Model file for the job. Use its own axes, mm. A direction names the side the tool comes from. Coordinates: 2 decimals unless noted, no trailing zeros. Order: outer loops, then holes, each group sorted by start corner. A loop starts at its lowest first (then second) coordinate and runs counter-clockwise, first axis right, second up.
from build123d import *

# Parameters (mm, degrees)
THICKNESS_EXTRUDE_DEPTH = 2
HOOK_1_EXTRUDE_DEPTH    = 0.9
HOOK_START              = -26.75
HOOK_2_EXTRUDE_DEPTH    = 0.9
HOOK_PATTERN_COUNT      = 2
HOOK_PATTERN_PITCH      = 96


with BuildPart() as part:
    # Top Sketch → Thickness Extrude (new body)
    with BuildSketch(Plane(origin=(0, 0, 0), x_dir=(1, 0, 0), z_dir=(0, 1, 0))):
        Polygon((-28, -21.5), (-28, -22.875), (-31, -22.875), (-31, -21.5), (-124, -21.5), (-124, -22.875), (-127, -22.875), (-127, -21.5), (-168, -21.5), (-168, 0), (-127, 0), (-127, 3.875), (-124, 3.875), (-124, 0), (-31, 0), (-31, 3.875), (-28, 3.875), (-28, 0), (0, 0), (0, -21.5), align=None)
    extrude(amount=THICKNESS_EXTRUDE_DEPTH)


with BuildPart() as body_2:
    # Hook Sketch → Hook 1 Extrude (new, symmetric)
    with BuildSketch(Plane.XY.offset(22.875)):
        Polygon((-31, 2), (-28, 2), (-28, -4.258262488), (-36, -4.258262488), (-36, -2.258262488), (-31, -1.6), align=None)
    hook_1_extrude = extrude(amount=HOOK_1_EXTRUDE_DEPTH, both=True)


with BuildPart() as body_3:
    # Hook Sketch<2> → Hook 2 Extrude (new, symmetric)
    with BuildSketch(Plane.XY.offset(22.875).offset(HOOK_START)):
        Polygon((-31, 2), (-28, 2), (-28, -4.258262488), (-36, -4.258262488), (-36, -2.258262488), (-31, -1.6), align=None)
    hook_2_extrude = extrude(amount=HOOK_2_EXTRUDE_DEPTH, both=True)


with BuildPart() as hook_pattern_1:
    # Hook Pattern: pattern copy
    add(hook_1_extrude.moved(Location(Vector(-1, 0, 0) * (1 * HOOK_PATTERN_PITCH))))


with BuildPart() as hook_pattern_2:
    # Hook Pattern: pattern copy
    add(hook_2_extrude.moved(Location(Vector(-1, 0, 0) * (1 * HOOK_PATTERN_PITCH))))


with BuildPart() as part_1:
    add(part.part)

    # Combine Bodies: union body 2, body 3, Hook Pattern_1, Hook Pattern_2
    add(body_2.part)
    add(body_3.part)
    add(hook_pattern_1.part)
    add(hook_pattern_2.part)


solid = part_1.part
Q1. Cut at A-A, the plane z = -1.5. List the corners of the cut face in (x, y).
Established:
outline: (-127, 0) - (-124, 0) - (-124, 2) - (-127, 2) - close; (-31, 0) - (-28, 0) - (-28, 2) - (-31, 2) - close
Q2. Cut at D-D, the plane z = 15. List the corners of the cut face in (x, y).
Established:
outline: (-168, 0) - (0, 0) - (0, 2) - (-168, 2) - close
Q3. Cut at B-B, the plane x = -32.5. List the corners of the cut face in (y, z) (3 decimals).
Established:
outline: (-4.258, -4.775) - (-1.797, -4.775) - (-1.797, -2.975) - (-4.258, -2.975) - close; (-4.258, 21.975) - (-1.797, 21.975) - (-1.797, 23.775) - (-4.258, 23.775) - close; (0, 0) - (2, 0) - (2, 21.5) - (0, 21.5) - close
Q4. Mould opens along Z. For faces 1 (the face through (-127, -2, 23.775)), 2 (the face through (-31, 1, -3)), 3 (the face through (-127, -3, -2.975)) say: pulls with the +Z half, pulls with the -Z half, needs draft (parallel to the pull), parting line crosses it, or undercut.
Established:
face 1: pulls with the +Z half
face 2: needs draft
face 3: undercut
Q5. Which spindle directions (+Z, -Z, +X, -X, +Y, -Y) get a long thin tool onto all of the face, cutting with end or side? Do faces 4 (the face through (-127, 1, -3)), 5 (the face through (-28, -0.4, -3.4)), 6 (the face through (-31, -3, 21.975)), 7 (the face through (-124, -0.4, -3.4)). Say none if no direction does.
Established:
face 4: -Z, -X, +Y
face 5: -Z, +X, +Y, -Y
face 6: +X, -X, -Y
face 7: -Z, +Y, -Y
Q6. Probe line 1 (X direction, y = 1, z = 22.25); line 2 (Z direction, x = -128.5, y = -2) (3 decimals); line 3 (Y direction, x = -129, z = 7.25). List the from-to ranges inside material, lowest first.
Established:
line 1: x = -127 to -124, -31 to -28
line 2: z = -4.775 to -2.975, 21.975 to 23.775
line 3: y = 0 to 2
Q7. Drop flat-ended pins along their axis: P1, Ø1, axis at x = -79, y = 1.5, coming from the -Z side; P2, Ø0.5, axis at y = -3.5, z = 22.5, coming from the -X side; P3, Ø3, axis at y = 0, z = -2.5, coming from the -X side; P4, Ø2, axis at y = 0.5, z = 15, coming from the +X side. Give the stop position or say it passes through.
Established:
P1: stops at z = 0
P2: stops at x = -132
P3: stops at x = -127
P4: stops at x = 0
Q8. Cut at C-C, the plane x = -103. List the corners of the cut face in (y, z).
Established:
outline: (0, 0) - (2, 0) - (2, 21.5) - (0, 21.5) - close
